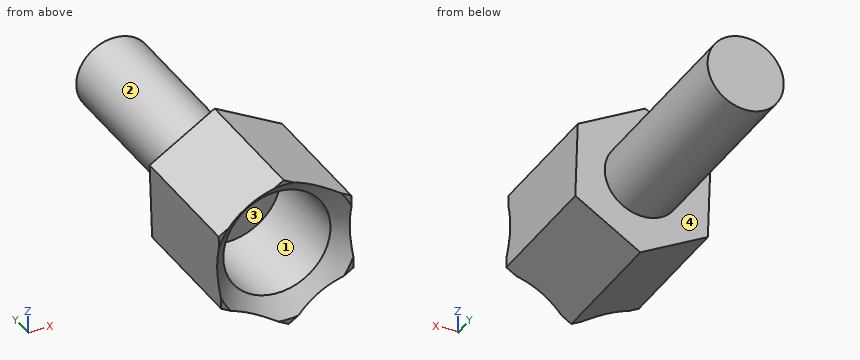
from build123d import *

# Parameters (mm, degrees)
EXTRUDE_1_DEPTH                 = 4.7
HOLE_WIZARD_10_24_1_D           = 3.7973
HOLE_WIZARD_10_24_1_DEPTH       = 4
HOLE_WIZARD_10_24_1_CSINK_D     = 5.0673
HOLE_WIZARD_10_24_1_CSINK_ANGLE = 90
SKETCH_5_R                      = 1.35
EXTRUDE_2_DEPTH                 = 7


with BuildPart() as part:
    # 草图1 → 凸台-拉伸1 (new body)
    with BuildSketch(Plane(origin=(0, 0, 0), x_dir=(1, 0, 0), z_dir=(0, 1, 0))):
        Polygon((2.304627048, -1.432489966), (2.392886225, 1.279620587), (0.088259177, 2.712110553), (-2.304627048, 1.432489966), (-2.392886225, -1.279620587), (-0.088259177, -2.712110553), align=None)
    extrude(amount=EXTRUDE_1_DEPTH)

    # #10-24 螺纹孔1
    with Locations(Plane.XZ):
        with Locations((0, 0)):
            CounterSinkHole(HOLE_WIZARD_10_24_1_D / 2, HOLE_WIZARD_10_24_1_CSINK_D / 2, depth=HOLE_WIZARD_10_24_1_DEPTH, counter_sink_angle=HOLE_WIZARD_10_24_1_CSINK_ANGLE)

    # 草图5 → 凸台-拉伸2 (add)
    with BuildSketch(Plane(origin=(0, 4.7, 0), x_dir=(-1, 0, 0), z_dir=(0, 1, 0))):
        with Locations(Location((0, 0, 0), (0, 0, 90))):
            Circle(SKETCH_5_R)
    extrude(amount=EXTRUDE_2_DEPTH)


solid = part.part
Verification items for the finished model (mm, model axes). Face numbers are marked on the shaded views. Give positions to 0.01 mm unless a question says otherwise; leave off trailing zeros. Loops run counter-clockwise (first coordinate to the right, second up) from the corner with the lowest first, then second, coordinate; pieces in that order, holes last. Notation, with made-up numbers: (-23, 1) - (26, 1) arc R21 ccw to (26, 15) - close; hole circle Ø8 at (-1.5, 19.25). An arc over 180 degrees is marked (long way). Write item = value, one per line. Start each with the question number.
Q1. Cross-section at A-A, the plane y = 4.25. Enter the section's corners in (x, z).
Q2. Depth check by flat-ended pin: P1, Ø1, axis at x = -1.5, y = 8, coming from the -Z side; P2, Ø1, axis at y = 6.5, z = 1.5, coming from the +X side; P3, Ø1, axis at x = -2, y = 5, coming from the +Z side. Enter the tip coordinate at first touch or a pass-through.
Q3. Thickness scan on line 1 (Y direction, x = 1.05, z = -0.35); line 2 (X direction, y = 2.6, z = 0); line 3 (Z direction, x = 0, y = 3.15). Record the ranges inside material, lowest first.
Q4. Cross-section at C-C, the plane y = 5.5. Enter the section's corners in (x, z).
Q5. Cross-section at B-B, the plane z = 0. Enter the section's corners in (x, y) (3 decimals).
Q6. Mould release check, pull along Z, two halves, no side actions. Record for the marked faces 1, 2, 3 and 4: released by +Z, released by -Z, zero draft, split by the parting line, or undercut.
Answer key:
q1.outline = (-2.39, 1.28) - (-2.3, -1.43) - (0.09, -2.71) - (2.39, -1.28) - (2.3, 1.43) - (-0.09, 2.71) - close
q2.P1 = -0.91
q2.P2 = 0.91
q2.P3 = 1.77
q3.line_1 = 4 to 11.7
q3.line_2 = -2.35 to -1.9, 1.9 to 2.35
q3.line_3 = -2.66 to -1.9, 1.9 to 2.66
q4.outline = circle Ø2.7 at (0, 0)
q5.outline = (-2.351, 0.182) - (-1.899, 0.635) - (-1.899, 4) - (1.899, 4) - (1.899, 0.635) - (2.351, 0.182) - (2.351, 4.7) - (1.35, 4.7) - (1.35, 11.7) - (-1.35, 11.7) - (-1.35, 4.7) - (-2.351, 4.7) - close
q6.face_1 = undercut
q6.face_2 = split by the parting line
q6.face_3 = undercut
q6.face_4 = zero draft
